Geometry check sheet. Reference: the model listing, model coordinates, mm. A direction names the side the tool comes from. Coordinates: 2 decimals unless noted, no trailing zeros. Write each loop counter-clockwise with the first axis right and the second up, starting at its lowest first coordinate (ties: lowest second). Pieces come first, ordered by that corner, then holes.
Autodesk Inventor part; units mm, degrees
ref_plane "YZ Plane" through (0, 0, 0) normal (1, 0, 0) x (0, 1, 0)
ref_plane "XZ Plane" through (0, 0, 0) normal (0, 1, 0) x (-1, 0, 0)
ref_plane "XY Plane" through (0, 0, 0) normal (0, 0, 1) x (1, 0, 0)
sketch "Sketch1" plane through (0, 0, 0) normal (0, 1, 0) x (-1, 0, 0)
  circle A0 centre (0, 0) radius 7.5
  circle A1 centre (0, 0) radius 1.5
  dimension "d0" = 15
  dimension "d1" = 3
extrude "Extrusion1" add sketch "Sketch1" along normal blind 15
thread "Thread1"
sketch "Sketch2" plane through (0, 15, 0) normal (0, 1, 0) x (1, 0, 0)
  circle A0 centre (0, 0) radius 4
  dimension "d6" = 8
extrude "Extrusion2" add sketch "Sketch2" along normal blind 15
loft "Loft1" add section 1 edges at (-4, 30, 0) section 2 edges at (7.5, 15, 0)
fillet "Fillet1" radius 4 1 edges at (-4, 30, 0)
properties part number "pull"
1. Access from +Z, -Z, +X, -X, +Y, -Y to the whole of each face (thin tool, end or side, straight path). Record for faces 4 (the cylindrical face through (7.493, 7.395, -0.33)), 5 (the cylindrical face through (1.5, 7.4, -0.07)).
Computed values:
face 4: +Y, -Y
face 5: -Y
2. Sectioned sample at A-A, the plane y = 14. Record the boundary of the cut face in (x, z), and give its area (3 significant figures).
Computed values:
outline: circle Ø15 at (0, 0); hole circle Ø3 at (0, 0)
area: 170 mm2
3. Draft check along X on faces 1 (the flat face through (0, 15, 0)), 2 (the conical face through (-1.262, 22.194, -5.683)), 3 (the flat face through (0, 0, -2)). Enter one of: released by +X, released by -X, zero draft, split by the parting line, or undercut.
Computed values:
face 1: undercut
face 2: split by the parting line
face 3: zero draft
4. Gauge pin test, flat ends, axial feed: pin 1 Ø5 at (y, z) = (24, -1.5) entering from +X; pin 2 Ø5 at (x, z) = (6, 2) entering from +Y; pin 3 Ø4 at (x, y) = (-3, 14.5) entering from -Z; pin 4 Ø5 at (y, z) = (17, 1) entering from -X. Record the tip position at first contact, or that the pin passes through.
Computed values:
pin 1: stops at x = 5.91
pin 2: stops at y = 28.65
pin 3: stops at z = -7.43
pin 4: stops at x = -7.5
5. Sectioned sample at C-C, the plane y = 19.5. Record the boundary of the cut face in (x, z), and give its area (3 significant figures).
Computed values:
outline: circle Ø12.9 at (0, 0)
area: 131 mm2
6. Sectioned sample at B-B, the plane y = 24. Record the boundary of the cut face in (x, z).
Computed values:
outline: circle Ø10.8 at (0, 0)
7. Thickness scan on line 1 along Z through (x, y) = (0, 5.5); line 2 along Z through (x, y) = (0.5, 12.5); line 3 along Y through (x, z) = (0.5, -0.5). Record the ranges inside material, lowest first.
Computed values:
line 1: z = -7.5 to -1.5, 1.5 to 7.5
line 2: z = -7.48 to -1.41, 1.41 to 7.48
line 3: y = 15 to 30
